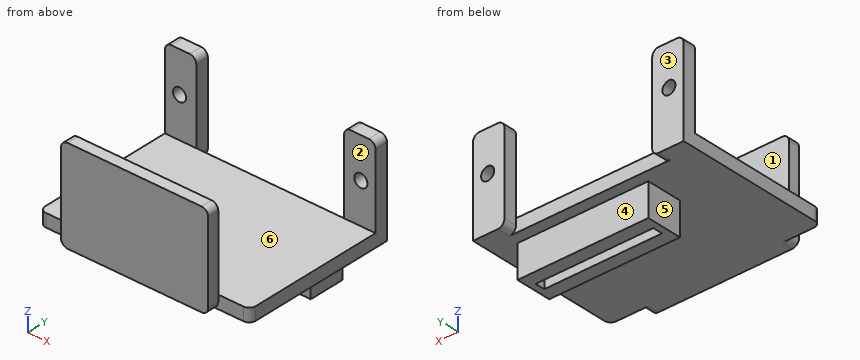
```python
from build123d import *

# Parameters (mm, degrees)
SKETCH1_W           = 32.2
SKETCH1_H           = 25.5
BOSS_EXTRUDE1_DEPTH = 14.4
SKETCH3_W           = 32.2
SKETCH3_H           = 21.75
CUT_EXTRUDE1_DEPTH  = 12.4
SKETCH5_W           = 22.6
SKETCH5_H           = 2
CUT_EXTRUDE2_DEPTH  = 14.4
FILLET1_R           = 1
FILLET2_R           = 1
FILLET3_R           = 1
FILLET4_R           = 1
SKETCH10_R          = 1
CUT_EXTRUDE3_DEPTH  = 10
SKETCH11_W          = 4.85
SKETCH11_H          = 1.75
CUT_EXTRUDE4_DEPTH  = 20
FILLET5_R           = 1
FILLET6_R           = 1
SKETCH12_W          = 20
SKETCH12_H          = 2
BOSS_EXTRUDE2_DEPTH = 5
BOSS_EXTRUDE3_DEPTH = 5


with BuildPart() as part:
    # Sketch1 → Boss-Extrude1 (new body)
    with BuildSketch(Plane.XY):
        Rectangle(SKETCH1_W, SKETCH1_H)
    extrude(amount=BOSS_EXTRUDE1_DEPTH)

    # Sketch3 → Cut-Extrude1 (cut)
    with BuildSketch(Plane.XY.offset(14.4)):
        with Locations((0, -0.125)):
            Rectangle(SKETCH3_W, SKETCH3_H)
    extrude(amount=-CUT_EXTRUDE1_DEPTH, mode=Mode.SUBTRACT)

    # Sketch5 → Cut-Extrude2 (cut)
    with BuildSketch(Plane.XY.offset(14.4)):
        with Locations((0, 11.75)):
            Rectangle(SKETCH5_W, SKETCH5_H)
    extrude(amount=-CUT_EXTRUDE2_DEPTH, mode=Mode.SUBTRACT)

    # Fillet1
    fillet1_edges = [part.edges().sort_by_distance(p)[0] for p in [
        (-11.3, 11.75, 14.4),
    ]]
    fillet(fillet1_edges, radius=FILLET1_R)

    # Fillet2
    fillet2_edges = [part.edges().sort_by_distance(p)[0] for p in [
        (-16.1, 11.75, 14.4),
    ]]
    fillet(fillet2_edges, radius=FILLET2_R)

    # Fillet3
    fillet3_edges = [part.edges().sort_by_distance(p)[0] for p in [
        (11.3, 11.75, 14.4),
    ]]
    fillet(fillet3_edges, radius=FILLET3_R)

    # Fillet4
    fillet4_edges = [part.edges().sort_by_distance(p)[0] for p in [
        (16.1, 11.75, 14.4),
    ]]
    fillet(fillet4_edges, radius=FILLET4_R)

    # Sketch10 → Cut-Extrude3 (cut)
    with BuildSketch(Plane(origin=(0, 12.75, 0), x_dir=(1, 0, 0), z_dir=(0, 1, 0))):
        with Locations(Location((-13.86, -8.203047487, 0), (0, 0, 270))):
            Circle(SKETCH10_R)
    cut_extrude3 = extrude(amount=-CUT_EXTRUDE3_DEPTH, mode=Mode.SUBTRACT)

    # Mirror1: Cut-Extrude3 across plane
    add(cut_extrude3.mirror(Plane(origin=(0, 0, 0), x_dir=(0, 0, 1), z_dir=(1, 0, 0))), mode=Mode.SUBTRACT)

    # Sketch11 → Cut-Extrude4 (cut)
    with BuildSketch(Plane.XY.offset(14.4)):
        with Locations((-13.675, -11.875)):
            Rectangle(SKETCH11_W, SKETCH11_H)
    cut_extrude4 = extrude(amount=-CUT_EXTRUDE4_DEPTH, mode=Mode.SUBTRACT)

    # Mirror2: Cut-Extrude4 across plane
    add(cut_extrude4.mirror(Plane(origin=(0, 0, 0), x_dir=(0, 0, 1), z_dir=(1, 0, 0))), mode=Mode.SUBTRACT)

    # Fillet5
    fillet5_edges = [part.edges().sort_by_distance(p)[0] for p in [
        (16.1, -11, 1),
        (11.25, -11.875, 14.4),
        (11.25, -11.875, 0),
        (-11.25, -11.875, 0),
        (-16.1, -11, 1),
        (-11.25, -11.875, 14.4),
    ]]
    fillet(fillet5_edges, radius=FILLET5_R)

    # Fillet6
    fillet6_edges = [part.edges().sort_by_distance(p)[0] for p in [
        (-11.3, 11.75, 0),
        (11.3, 11.75, 0),
    ]]
    fillet(fillet6_edges, radius=FILLET6_R)

    # Sketch12 → Boss-Extrude2 (add)
    with BuildSketch(Plane(origin=(0, 0, 0), x_dir=(-1, 0, 0), z_dir=(0, 0, -1))):
        with Locations((-2.6, 4.5)):
            Rectangle(SKETCH12_W, SKETCH12_H)
    extrude(amount=BOSS_EXTRUDE2_DEPTH)

    # Sketch13 → Boss-Extrude3 (add)
    with BuildSketch(Plane(origin=(0, 0, 0), x_dir=(-1, 0, 0), z_dir=(0, 0, -1))):
        Polygon((-12.6, 9), (7.4, 9), (7.4, 7), (7.4, 5.5), (6.4, 5.5), (6.4, 7), (-11.6, 7), (-11.6, 5.5), (-12.6, 5.5), (-12.6, 7), align=None)
    extrude(amount=BOSS_EXTRUDE3_DEPTH)


solid = part.part
```
Geometry check sheet. Reference: the model listing, model coordinates, mm. Face numbers are marked on the shaded views. A direction names the side the tool comes from. Coordinates: 2 decimals unless noted, no trailing zeros. Write each loop counter-clockwise with the first axis right and the second up, starting at its lowest first coordinate (ties: lowest second). Pieces come first, ordered by that corner, then holes. Notation, with made-up numbers: M 2,-37.75 L 54,-37.75 A24 cw 54,-27.75 Z; hole C 64.5,82.25 d8. An arc over 180 degrees is marked long. Use one line per item in the form item = value. Start each with the question number.
1) Section check D-D on z = 12.5. Enter the section's corners in (x, y), and give its area (3 significant figures).
2) Section check B-B on z = -0.5. Enter the section's corners in (x, y), and give its area (3 significant figures).
3) Release check for a two-part mould opening along X. For the marked faces 5 and 6 record: pulls with the +X half, pulls with the -X half, needs draft (parallel to the pull), parting line crosses it, or undercut.
4) Section check C-C on y = 4.5. Enter the section's corners in (x, z).
5) Section check A-A on x = 13.86. Enter the section's corners in (y, z), and give its area (3 significant figures).
6) Go/stop test with flat-tipped pins: pin 1 Ø0.6 at (x, z) = (-1, 0.5) entering from +Y; pin 2 Ø3.5 at (x, z) = (2.5, 10.5) entering from +Y; pin 3 Ø0.8 at (x, y) = (4.5, 6) entering from -Z. Record where each tip stops, or that it passes through.
7) Thickness scan on probe 1 along Y at (x, z) = (-3.5, -2.25); probe 2 along X at (y, z) = (11.5, 12); probe 3 along Z at (x, y) = (8, 3). Record the ranges inside material, lowest first. Write a range as from..to.
8) Set-up check for the marked faces 1, 2, 3 and 4: record each of +Z, -Z, +X, -X, +Y, -Y from which the full face is reachable in a straight line by a thin tool's end or side.
Responses:
q1.outline = M -16.1,10.75 L -11.3,10.75 L -11.3,12.75 L -16.1,12.75 Z; M -11.25,-12.75 L 11.25,-12.75 L 11.25,-11 L -11.25,-11 Z; M 11.3,10.75 L 16.1,10.75 L 16.1,12.75 L 11.3,12.75 Z
q1.area = 58.6 mm2
q2.outline = M -7.4,3.5 L 12.6,3.5 L 12.6,9 L -7.4,9 Z; hole M -6.4,5.5 L 11.6,5.5 L 11.6,7 L -6.4,7 Z
q2.area = 83.0 mm2
q3.face_5 = pulls with the -X half
q3.face_6 = needs draft
q4.outline = M -16.1,0 L -7.4,0 L -7.4,-5 L 12.6,-5 L 12.6,0 L 16.1,0 L 16.1,2 L -16.1,2 Z
q5.outline = M -11,0 L 12.75,0 L 12.75,7.2 L 10.75,7.2 L 10.75,2 L -11,2 Z; M 10.75,9.2 L 12.75,9.2 L 12.75,14.4 L 10.75,14.4 Z
q5.area = 68.3 mm2
q6.pin_1 = 10.75
q6.pin_2 = -11
q6.pin_3 = 0
q7.probe_1 = 3.5..5.5, 7..9
q7.probe_2 = -16.1..-11.3, 11.3..16.1
q7.probe_3 = 0..2
q8.face_1 = +Z, +X, -X, +Y
q8.face_2 = +Z, +X, -X, -Y
q8.face_3 = +Z, -Z, +X, -X, +Y
q8.face_4 = -Z, +X, -X, +Y
